CAD build for the part. Positions are in the model's coordinates, mm. Face numbers are marked on the shaded views. A direction names the side the tool comes from. Round coordinates to 2 decimals unless told otherwise and drop trailing zeros. Write each loop counter-clockwise with the first axis right and the second up, starting at its lowest first coordinate (ties: lowest second). Pieces come first, ordered by that corner, then holes. Notation, with made-up numbers: (3.25, 22) - (26.25, 22) arc R19 ccw to (26.25, 38) - close; hole circle Ø9 at (82, 58.5). An arc over 180 degrees is marked (long way). Answer in a Markdown table with one row per item.
```python
from build123d import *

# Parameters (mm, degrees)
SKETCH1_R                 = 38.1
MAIN_BODY_DEPTH           = 27.94
SKETCH2_R                 = 17.5
STATIC_SEAL_HOLE_DEPTH    = 10.25
SHAFT_HOLE_D              = 18
SKETCH14_R                = 38.1
SKETCH14_R_2              = 22.225
ROTATING_SEAL_SPACE_DEPTH = 25.4
FACE_START                = -6.35
SKETCH7_R                 = 50.8
SKETCH7_R_2               = 22.225
FACE_JOINT_DEPTH          = 6.35
SKETCH8_R                 = 20
BEARING_HOLE_DEPTH        = 13
SCREW_HOLES_D             = 10
SKETCH16_R                = 32.7406
SKETCH16_R_2              = 28.575
GASKET_RING_DEPTH         = 1.27


with BuildPart() as part:
    # Sketch1 → main body (new body)
    with BuildSketch(Plane(origin=(0, 0, 0), x_dir=(0, 0, -1), z_dir=(1, 0, 0))):
        Circle(SKETCH1_R)
    extrude(amount=MAIN_BODY_DEPTH)

    # Sketch2 → Static Seal Hole (cut)
    with BuildSketch(Plane(origin=(27.94, 0, 0), x_dir=(0, 0, -1), z_dir=(1, 0, 0))):
        Circle(SKETCH2_R)
    extrude(amount=-STATIC_SEAL_HOLE_DEPTH, mode=Mode.SUBTRACT)

    # Shaft hole (through all)
    with Locations(Plane(origin=(17.69, 0, 0), x_dir=(0, 0, -1), z_dir=(1, 0, 0))):
        with Locations((0, 0)):
            Hole(SHAFT_HOLE_D / 2)

    # Sketch14 → rotating seal space (add)
    with BuildSketch(Plane(origin=(27.94, 0, 0), x_dir=(0, 0, -1), z_dir=(1, 0, 0))):
        Circle(SKETCH14_R)
        Circle(SKETCH14_R_2, mode=Mode.SUBTRACT)
    extrude(amount=ROTATING_SEAL_SPACE_DEPTH)

    # Sketch7 → face joint (add)
    with BuildSketch(Plane(origin=(53.34, 0, 0), x_dir=(0, 0, -1), z_dir=(1, 0, 0)).offset(FACE_START)):
        Circle(SKETCH7_R)
        Circle(SKETCH7_R_2, mode=Mode.SUBTRACT)
    extrude(amount=FACE_JOINT_DEPTH)

    # Sketch8 → bearing hole (cut)
    with BuildSketch(Plane.ZY):
        Circle(SKETCH8_R)
    extrude(amount=-BEARING_HOLE_DEPTH, mode=Mode.SUBTRACT)

    # Screw holes (through all)
    with Locations(Plane.ZY.offset(-46.99)):
        with Locations((-44.206688043, 0), (-31.258848889, 31.258848889), (0, 44.206688043), (31.258848889, 31.258848889), (44.206688043, 0), (31.258848889, -31.258848889), (0, -44.206688043), (-31.258848889, -31.258848889), (0, 0)):
            Hole(SCREW_HOLES_D / 2)

    # Sketch16 → Gasket ring (cut)
    with BuildSketch(Plane(origin=(53.34, 0, 0), x_dir=(0, 0, -1), z_dir=(1, 0, 0))):
        Circle(SKETCH16_R)
        Circle(SKETCH16_R_2, mode=Mode.SUBTRACT)
    extrude(amount=-GASKET_RING_DEPTH, mode=Mode.SUBTRACT)


solid = part.part
```
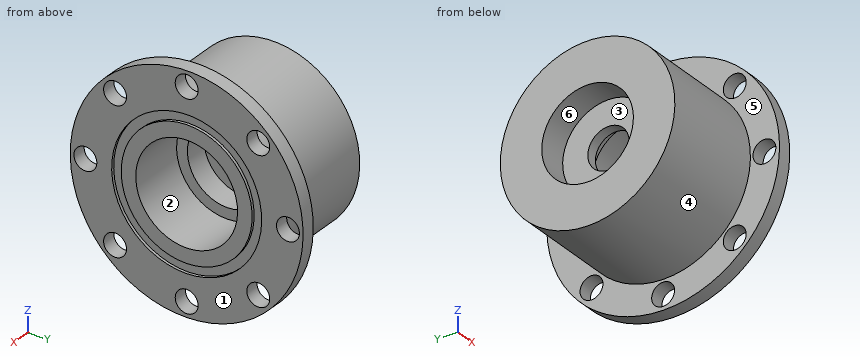
Q1. Drill centre lines: line 1 (Y direction, x = 51, z = 0) (3 decimals); line 2 (Y direction, x = 23.75, z = 0); line 3 (X direction, y = 38, z = 26). Where is each one in solid material? Low to high.
Computed:
| item | result |
|---|---|
| line 1 | y = -50.8 to -49.207, -39.207 to -22.225, 22.225 to 39.207, 49.207 to 50.8 |
| line 2 | y = -38.1 to -17.5, 17.5 to 38.1 |
| line 3 | x = 46.99 to 53.34 |
Q2. Saw through at A-A on z = 43.5. List the corners of the cut face in (x, y), then the cut area to 3 significant figures.
Computed:
| item | result |
|---|---|
| outline | (46.99, -26.24) - (53.34, -26.24) - (53.34, -4.95) - (46.99, -4.95) - close; (46.99, 4.95) - (53.34, 4.95) - (53.34, 26.24) - (46.99, 26.24) - close |
| area | 270 mm2 |
Q3. 3-axis set-ups, long thin cutter, end or side, ignore diameter. For the marked faces 1, 2 and 3: which of +Z, -Z, +X, -X, +Y, -Y reach the whole face in a straight line?
Computed:
| item | result |
|---|---|
| face 1 | +Z, -Z, +X, +Y, -Y |
| face 2 | +X |
| face 3 | -X |
Q4. Flat gauge pins, fed straight in: pin 1 (17.5 mm diameter, centred on y = 5.5, z = -3.5, fed in from +X); pin 2 (12 mm diameter, centred on x = 28.5, z = 12.5, fed in from +Y); pin 3 (8 mm diameter, centred on x = 44, z = 7, fed in from +Y). Where does each tip first touch, or does it go through?
Computed:
| item | result |
|---|---|
| pin 1 | stops at x = 17.69 |
| pin 2 | stops at y = 37.54 |
| pin 3 | stops at y = 50.61 |
Q5. Saw through at B-B on z = 0. Count the separate pieces of the cut face and the enclosed holes in it, then the cut area to 3 significant figures.
Computed:
| item | result |
|---|---|
| separate pieces | 4 |
| enclosed holes | 0 |
| area | 2,000 mm2 |
Q6. Pull direction Y, two halves, no side cores. Call the marked faces 4, 5 and 6: released by +Y, released by -Y, zero draft, split by the parting line, or undercut.
Computed:
| item | result |
|---|---|
| face 4 | split by the parting line |
| face 5 | zero draft |
| face 6 | undercut |
Q7. Saw through at D-D on z = -14. List the corners of the cut face in (x, y).
Computed:
| item | result |
|---|---|
| outline | (0, -35.43) - (46.99, -35.43) - (46.99, -48.83) - (53.34, -48.83) - (53.34, -29.6) - (52.07, -29.6) - (52.07, -24.91) - (53.34, -24.91) - (53.34, -17.26) - (27.94, -17.26) - (27.94, -10.5) - (17.69, -10.5) - (17.69, 10.5) - (27.94, 10.5) - (27.94, 17.26) - (53.34, 17.26) - (53.34, 24.91) - (52.07, 24.91) - (52.07, 29.6) - (53.34, 29.6) - (53.34, 48.83) - (46.99, 48.83) - (46.99, 35.43) - (0, 35.43) - (0, 14.28) - (13, 14.28) - (13, -14.28) - (0, -14.28) - close |
